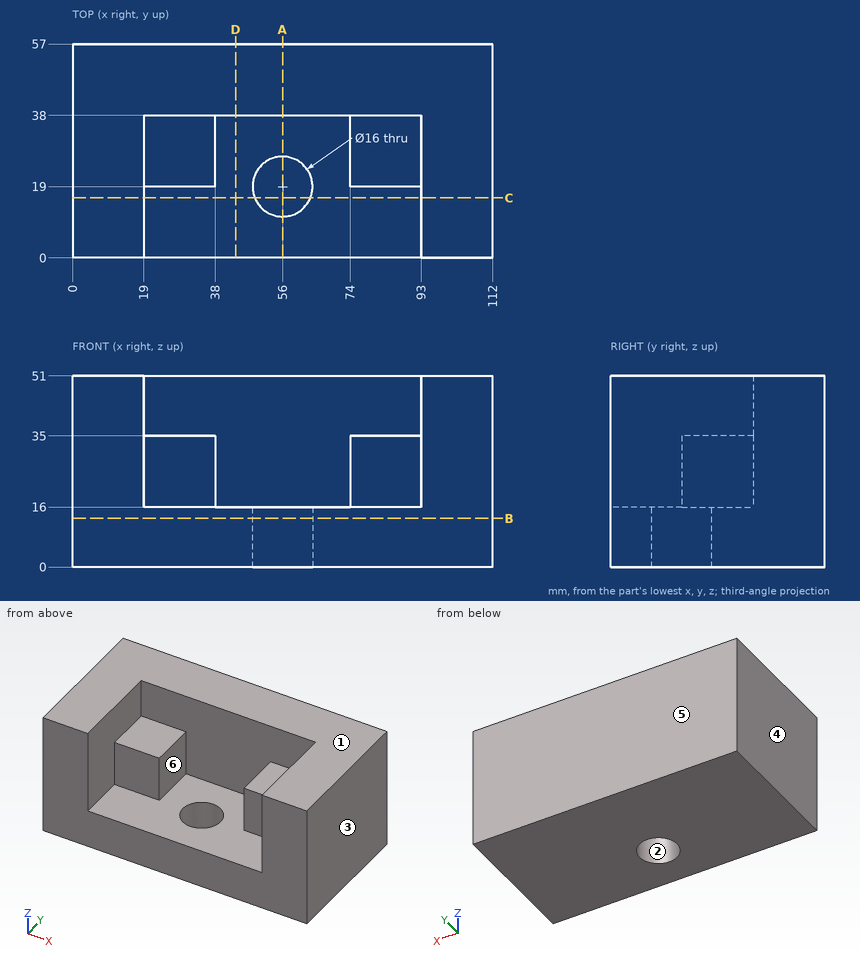
Answer from the drawing. Dimensions are ordinates in mm from the lowest x, y and z of the part. A direction names the side the tool comes from. Coordinates: 2 decimals unless noted, no trailing zeros. Write each loop counter-clockwise with the first axis right and the second up, starting at its lowest first coordinate (ties: lowest second). Pieces come first, ordered by that corner, then holes. Notation, with made-up numbers: M -36,21 L -21,21 A31 ccw -21,50 Z; hole C -5.5,-39.75 d9. An arc over 180 degrees is marked long. Put each result on its own line as item: value. Start each with the question number.
1. A cutting plane is placed at D-D on x = 43.5. Write down the section's boundary in (y, z).
2. A cutting plane is placed at A-A on x = 56. Write down the section's boundary in (y, z), then the cut area to 3 significant figures.
3. For a pull along X with two mould halves and no side action, classify the marked faces 1, 2, 3 and 4 as pulls with the +X half, pulls with the -X half, needs draft (parallel to the pull), parting line crosses it, or undercut.
4. Flat-ended cylindrical pins translate along their axes: P1, Ø2, axis at x = 40.5, y = 20, coming from the +Z side; P2, Ø5.5, axis at x = 80, y = 29, coming from the +Z side; P3, Ø9.5, axis at x = 29.5, z = 29, coming from the -Y side. Find the tip coordinate at first contact, or state that the pin passes through.
5. Which of the six approach directions +Z, -Z, +X, -X, +Y, -Y give full straight-line access (tool end or side, diameter ignored) to the marked faces 5 and 6?
6. A cutting plane is placed at B-B on z = 13. Write down the section's boundary in (x, y), then the cut area to 3 significant figures.
7. A cutting plane is placed at C-C on y = 16. Write down the section's boundary in (x, z).
8. Consider line 1 (Y direction, x = 56, z = 6.25); line 2 (X direction, y = 27.5, z = 17.5); line 3 (X direction, y = 14.5, z = 42). Determine where each line is inside the solid, lowest interval first. Write a range as from..to.
Resolved:
1. outline: M 0,0 L 57,0 L 57,51 L 38,51 L 38,16 L 0,16 Z
2. outline: M 0,0 L 11,0 L 11,16 L 0,16 Z; M 27,0 L 57,0 L 57,51 L 38,51 L 38,16 L 27,16 Z
2. area: 1,320 mm2
3. face 1: needs draft
3. face 2: undercut
3. face 3: pulls with the +X half
3. face 4: pulls with the -X half
4. P1: stops at z = 16
4. P2: stops at z = 35
4. P3: stops at y = 19
5. face 5: +Z, -Z, +X, -X, +Y
5. face 6: +Z, -Y
6. outline: M 0,0 L 112,0 L 112,57 L 0,57 Z; hole C 56,19 d16
6. area: 6,180 mm2
7. outline: M 0,0 L 48.58,0 L 48.58,16 L 19,16 L 19,51 L 0,51 Z; M 63.42,0 L 112,0 L 112,51 L 93,51 L 93,16 L 63.42,16 Z
8. line 1: y = 0..11, 27..57
8. line 2: x = 0..38, 74..112
8. line 3: x = 0..19, 93..112
